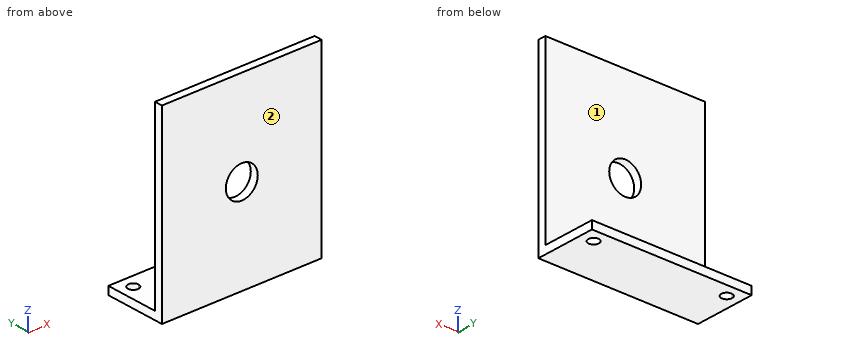
```python
from build123d import *

# Parameters (mm, degrees)
F0_W     = 60
F0_H     = 70
F1_DEPTH = 3
F2_W     = 60
F2_H     = 3
F3_DEPTH = 20
F5_DEPTH = 3
F6_R     = 6
F7_DEPTH = 3


with BuildPart() as f1:
    # F0 (on Front) → F1 (new body)
    with BuildSketch(Plane.XZ):
        Rectangle(F0_W, F0_H)
    extrude(amount=F1_DEPTH)

    # F2 (on face) → F3 (join)
    with BuildSketch(Plane(origin=(0, 0, 0), x_dir=(-1, 0, 0), z_dir=(0, 1, 0))):
        with Locations((0, -33.5)):
            Rectangle(F2_W, F2_H)
    extrude(amount=F3_DEPTH)

    # F4 (on face) → F5 (cut)
    with BuildSketch(Plane.XY.offset(-32)):
        with BuildLine():
            ThreePointArc((26.997119, 15.00453), (22.99712, 15.006795), (26.997114, 15))
            ThreePointArc((26.997114, 15), (26.997118, 15.002265), (26.997119, 15.00453))
        make_face()
        with BuildLine():
            ThreePointArc((-23.012635, 15.008898), (-25.017084, 17.008893), (-27.012615, 15))
            ThreePointArc((-27.012615, 15), (-25.008186, 13.008903), (-23.012635, 15.008898))
        make_face()
    extrude(amount=-F5_DEPTH, mode=Mode.SUBTRACT)

    # F6 (on face) → F7 (cut)
    with BuildSketch(Plane.XZ.offset(3)):
        Circle(F6_R)
    extrude(amount=-F7_DEPTH, mode=Mode.SUBTRACT)


solid = f1.part
```
Geometry check sheet. Reference: the model listing, model coordinates, mm. Face numbers are marked on the shaded views. A direction names the side the tool comes from. Round coordinates to 2 decimals unless told otherwise and drop trailing zeros. Write each loop counter-clockwise with the first axis right and the second up, starting at its lowest first coordinate (ties: lowest second). Pieces come first, ordered by that corner, then holes. Notation, with made-up numbers: (-32.75, -18.5) - (13.25, -18.5) arc R22 ccw to (13.25, 13.5) - close; hole circle Ø11 at (64.25, 29). An arc over 180 degrees is marked (long way). Write each question's results on one line, items separated by ' | '.
(1) Sectioned sample at C-C, the plane y = 4. Enter the section's corners in (x, z).
Computed:
outline: (-30, -35) - (30, -35) - (30, -32) - (-30, -32) - close
(2) Sectioned sample at B-B, the plane x = 0. Enter the section's corners in (y, z), plus the area to 3 significant figures.
Computed:
outline: (-3, -35) - (20, -35) - (20, -32) - (0, -32) - (0, -6) - (-3, -6) - close; (-3, 6) - (0, 6) - (0, 35) - (-3, 35) - close | area: 234 mm^2
(3) Sectioned sample at D-D, the plane x = 19. Enter the section's corners in (y, z).
Computed:
outline: (-3, -35) - (20, -35) - (20, -32) - (0, -32) - (0, 35) - (-3, 35) - close
(4) Sectioned sample at A-A, the plane z = 0. Enter the section's corners in (x, y).
Computed:
outline: (-30, -3) - (-6, -3) - (-6, 0) - (-30, 0) - close; (6, -3) - (30, -3) - (30, 0) - (6, 0) - close
(5) Depth check by flat-ended pin: pin 1 Ø6 at (x, y) = (-10, 6) entering from +Z; pin 2 Ø3 at (x, y) = (25, 15) entering from -Z (3 decimals); pin 3 Ø3 at (x, z) = (11, 25.5) entering from +Y. Enter the tip coordinate at first touch or a pass-through.
Computed:
pin 1: stops at z = -32 | pin 2: passes through | pin 3: stops at y = 0
(6) Set-up check for the marked faces 1 and 2: record each of +Z, -Z, +X, -X, +Y, -Y from which the full face is reachable in a straight line by a thin tool's end or side.
Computed:
face 1: +Z, +X, -X, +Y | face 2: +Z, -Z, +X, -X, -Y
(7) Thickness scan on probe 1 along Z at (x, y) = (0, -1.05); probe 2 along Z at (x, y) = (9, 8); probe 3 along Y at (x, z) = (-20, 3.5). Record the ranges inside material, lowest first. Write a range as from..to.
Computed:
probe 1: z = -35..-6, 6..35 | probe 2: z = -35..-32 | probe 3: y = -3..0
